Part print with two shaded views. Sizes in mm from the minimum x, y, z corner. Round coordinates to 2 decimals unless told otherwise and drop trailing zeros. Loops run counter-clockwise (first coordinate to the right, second up) from the corner with the lowest first, then second, coordinate; pieces in that order, holes last. Notation, with made-up numbers: (80, -27) -> (130, -27) arc R31 ccw to (130, 9) -> close; hole circle Ø5 at (-17.5, 2.25). An arc over 180 degrees is marked (long way). Use a Markdown table: item, result. Add a question column.
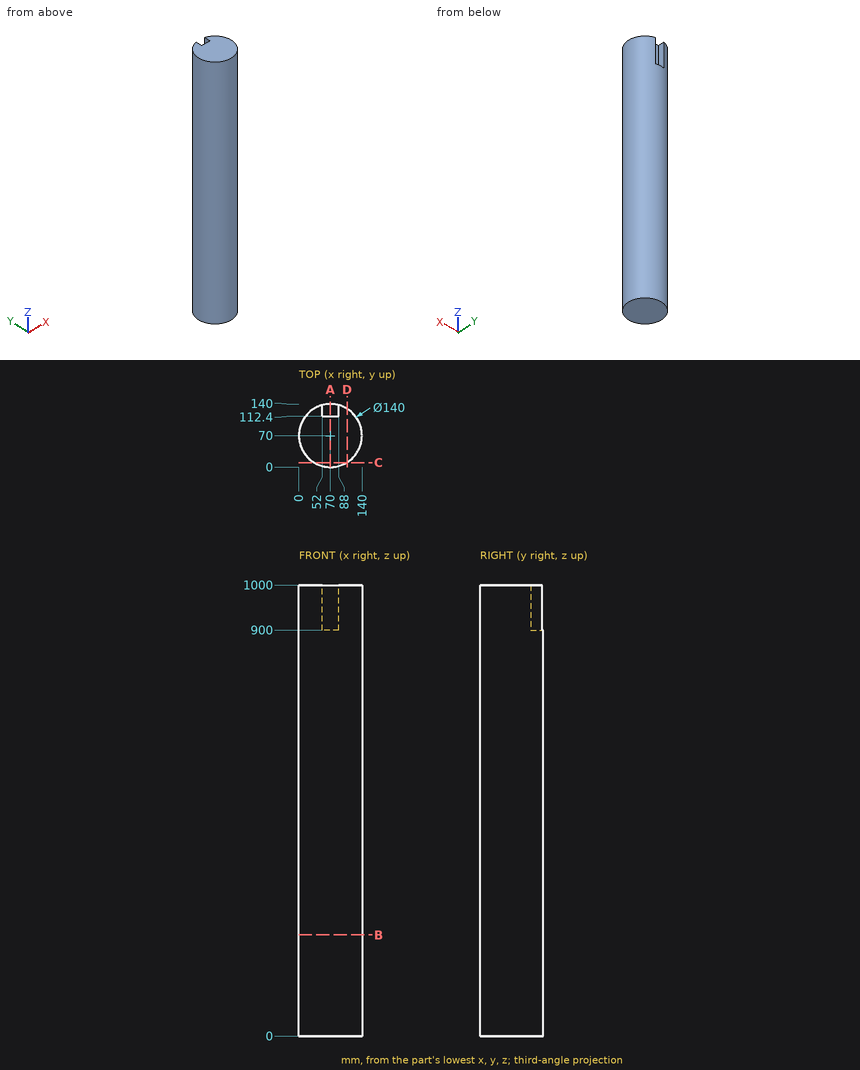
1) Cut at B-B on z = 224.5. Write the cut outline in (x, y), and give its area (3 significant figures).
2) Pin check, flat tips, straight feed: pin 1 Ø10 at (y, z) = (55.5, 239.5) entering from +X; pin 2 Ø12.5 at (y, z) = (122.5, 941.5) entering from -X; pin 3 Ø4 at (x, y) = (66.5, 125.5) entering from +Z. Stop position of each tip, or through.
3) Wall check: probe 1 along X at (y, z) = (67, 446.5); probe 2 along Y at (x, z) = (66, 123); probe 3 along Y at (x, z) = (72, 195). Give the ranges that are in metal, low to high. Write a range as from..to.
4) Cut at C-C on y = 10. Write the cut outline in (x, z), and give its area (3 significant figures).
5) Cut at A-A on x = 70. Write the cut outline in (y, z), and give its area (3 significant figures).
6) Cut at D-D on x = 107. Write the cut outline in (y, z), and give its area (3 significant figures).
Established:
| question | item | result |
|---|---|---|
| 1 | outline | circle Ø140 at (70, 70) |
| 1 | area | 15,400 mm^2 |
| 2 | pin 1 | stops at x = 139.35 |
| 2 | pin 2 | stops at x = 17.46 |
| 2 | pin 3 | stops at z = 900 |
| 3 | probe 1 | x = 0.06..139.94 |
| 3 | probe 2 | y = 0.11..139.89 |
| 3 | probe 3 | y = 0.03..139.97 |
| 4 | outline | (33.94, 0) -> (106.06, 0) -> (106.06, 1000) -> (33.94, 1000) -> close |
| 4 | area | 72,100 mm^2 |
| 5 | outline | (0, 0) -> (140, 0) -> (140, 900) -> (112.4, 900) -> (112.4, 1000) -> (0, 1000) -> close |
| 5 | area | 137,000 mm^2 |
| 6 | outline | (10.58, 0) -> (129.42, 0) -> (129.42, 1000) -> (10.58, 1000) -> close |
| 6 | area | 119,000 mm^2 |
